Could you check a few things on this model? Use its own coordinates, in mm. A direction names the side the tool comes from. Round coordinates to 2 decimals unless told otherwise and drop trailing zeros. Write each loop counter-clockwise with the first axis right and the second up, starting at its lowest first coordinate (ties: lowest second). Pieces come first, ordered by that corner, then holes. Notation, with made-up numbers: (-7, -6) -> (1, -6) arc R13 ccw to (1, 17) -> close; hole circle Ø11 at (56.25, 2.25). An arc over 180 degrees is marked (long way). Answer in a Markdown table with one row per item. Add a question column.
```python
from build123d import *

# Parameters (mm, degrees)
SKETCH1_W           = 125
SKETCH1_H           = 160
BOSS_EXTRUDE1_DEPTH = 60
SHELL1_T            = -10
CUT_EXTRUDE1_DEPTH  = 7


with BuildPart() as part:
    # Sketch1 → Boss-Extrude1 (new body)
    with BuildSketch(Plane(origin=(0, 0, 0), x_dir=(1, 0, 0), z_dir=(0, 1, 0))):
        Rectangle(SKETCH1_W, SKETCH1_H)
    extrude(amount=BOSS_EXTRUDE1_DEPTH)

    # Shell1
    shell1_openings = [part.faces().sort_by_distance(p)[0] for p in [
        (0, 60, 0),
        (0, 30, 80),
    ]]
    offset(amount=SHELL1_T, openings=shell1_openings, kind=Kind.INTERSECTION)

    # Sketch2 → Cut-Extrude1 (cut)
    with BuildSketch(Plane(origin=(0, 0, -80), x_dir=(-1, 0, 0), z_dir=(0, 0, -1))):
        with BuildLine():
            Line((58.149914344, 28.0000547), (-53.250098626, 28.0000547))
            ThreePointArc((-53.250098626, 28.0000547), (-59.250098626, 22.0000547), (-53.250098626, 16.0000547))
            Line((-53.250098626, 16.0000547), (58.149914344, 16.000100476))
            ThreePointArc((58.149914344, 16.000100476), (64.149891456, 22.000077588), (58.149914344, 28.0000547))
        make_face()
    extrude(amount=-CUT_EXTRUDE1_DEPTH, mode=Mode.SUBTRACT)


solid = part.part
```
(1) I need wall thicknesses on L1, parallel to X at y = 24.5, z = -41; L2, parallel to Y at x = -46.5, z = 65.5; L3, parallel to Z at x = -48.5, y = 52. Which ranges of each line are inside material? Lowest first, please.
(2) Suppose I cut it at C-C, the plane x = 10. Please give me the cut outline in (y, z), then the cut area to 3 significant figures.
(3) Suppose I cut it at A-A, the plane z = 67. Please give me the cut outline in (x, y), then the cut area to 3 significant figures.
(4) On a 3-axis mill with a long thin cutter (end or side, diameter ignored), from which of +Z, -Z, +X, -X, +Y, -Y can I reach the whole of each face in a straight line? I mean faces 4 (the face through (-3, 28, -77)), 5 (the face through (-62.5, 30, 1)), 6 (the face through (-52.5, 35, 6)). Say none if no direction works.
(5) For P1, Ø4, axis at x = 4, y = 13, coming from the +Z side; P2, Ø12, axis at x = 27, y = 21.5, coming from the -Z side; P3, Ø1.5, axis at x = -36, z = -26.5, coming from the +Y side, each with a flat end and sliding along its axis, tell me the tip position at first contact or that it passes through.
(6) If we mould it in two halves opening along Y, with no side actions, what happens to faces 1 (the face through (-60.486, 16.473, -76.549)), 2 (the face through (-1, 35, -70)), 3 (the face through (-1, 10, 4))? For each: pulls with the +Y half, pulls with the -Y half, needs draft (parallel to the pull), parting line crosses it, or undercut.
(7) Suppose I cut it at B-B, the plane y = 56. Please give me the cut outline in (x, z), then the cut area to 3 significant figures.
Response:
| question | item | result |
|---|---|---|
| 1 | L1 | -62.5 to -52.5, 52.5 to 62.5 |
| 1 | L2 | 0 to 10 |
| 1 | L3 | -80 to -70 |
| 2 | outline | (0, -80) -> (16, -80) -> (16, -73) -> (28, -73) -> (28, -80) -> (60, -80) -> (60, -70) -> (10, -70) -> (10, 80) -> (0, 80) -> close |
| 2 | area | 2,020 mm² |
| 3 | outline | (-62.5, 0) -> (62.5, 0) -> (62.5, 60) -> (52.5, 60) -> (52.5, 10) -> (-52.5, 10) -> (-52.5, 60) -> (-62.5, 60) -> close |
| 3 | area | 2,250 mm² |
| 4 | face 4 | -Z |
| 4 | face 5 | +Z, -Z, -X, +Y, -Y |
| 4 | face 6 | +Z, +Y |
| 5 | P1 | z = -70 |
| 5 | P2 | z = -80 |
| 5 | P3 | y = 10 |
| 6 | face 1 | undercut |
| 6 | face 2 | needs draft |
| 6 | face 3 | pulls with the +Y half |
| 7 | outline | (-62.5, -80) -> (62.5, -80) -> (62.5, 80) -> (52.5, 80) -> (52.5, -70) -> (-52.5, -70) -> (-52.5, 80) -> (-62.5, 80) -> close |
| 7 | area | 4,250 mm² |
